Design review of the part built by this model. Coordinates are the model's own, in mm. Coordinates: 2 decimals unless noted, no trailing zeros. Write each loop counter-clockwise with the first axis right and the second up, starting at its lowest first coordinate (ties: lowest second). Pieces come first, ordered by that corner, then holes.
Q1. Take a section at B-B (y = -13.75). Give the boundary of the cut face in (x, z) (3 decimals), and give its area (3 significant figures).
Q2. Insertion check: pin 1 (10 mm diameter, centred on x = -0.5, y = -9.5, fed in from +Z). The pin has a flat end and moves straight along its axis. Give the tip position at first contact, or say it passes through.
Q3. Take a section at A-A (z = -18). Give the boundary of the cut face in (x, y) (3 decimals), and give its area (3 significant figures).
Q4. For probe 1 along X at (y, z) = (-3.5, 18) (3 decimals); probe 2 along Z at (x, y) = (0, -4); probe 3 along X at (y, z) = (-9.5, 34) (3 decimals), list the stretches that pass through material, from the lowest coordinate up.
Q5. Take a section at C-C (x = 0). Give the boundary of the cut face in (y, z).
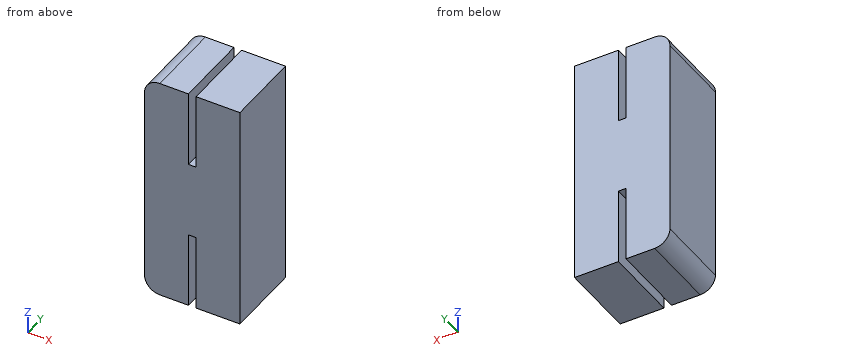
```python
from build123d import *

# Parameters (mm, degrees)
F0_W     = 31.75
F0_H     = 76.2
F1_DEPTH = 25.4
F2_W     = 2.54
F2_H     = 25.4
F3_DEPTH = 25.4
F4_R     = 5.08


with BuildPart() as f1:
    # F0 (on Front) → F1 (new body)
    with BuildSketch(Plane.XZ):
        Rectangle(F0_W, F0_H)
    extrude(amount=F1_DEPTH)

    # F2 (on face) → F3 (cut)
    with BuildSketch(Plane.XZ.offset(25.4)):
        with Locations((0, 25.4)):
            Rectangle(F2_W, F2_H)
        with Locations((0, -25.4)):
            Rectangle(F2_W, F2_H)
    extrude(amount=-F3_DEPTH, mode=Mode.SUBTRACT)

    # F4
    f4_edges = [f1.edges().sort_by_distance(p)[0] for p in [
        (-15.875, -12.7, 38.1),
        (-15.875, -12.7, -38.1),
    ]]
    fillet(f4_edges, radius=F4_R)


solid = f1.part
```
Response:
1. outline: (-15.875, -33.02) arc R5.08 ccw to (-10.795, -38.1) - (-1.27, -38.1) - (-1.27, -12.7) - (1.27, -12.7) - (1.27, -38.1) - (15.875, -38.1) - (15.875, 38.1) - (1.27, 38.1) - (1.27, 12.7) - (-1.27, 12.7) - (-1.27, 38.1) - (-10.795, 38.1) arc R5.08 ccw to (-15.875, 33.02) - close
1. area: 2,280 mm2
2. pin 1: stops at z = 38.1
3. outline: (-15.875, -25.4) - (-1.27, -25.4) - (-1.27, 0) - (-15.875, 0) - close; (1.27, -25.4) - (15.875, -25.4) - (15.875, 0) - (1.27, 0) - close
3. area: 742 mm2
4. probe 1: x = -15.875 to -1.27, 1.27 to 15.875
4. probe 2: z = -12.7 to 12.7
4. probe 3: x = -15.78 to -1.27, 1.27 to 15.875
5. outline: (-25.4, -12.7) - (0, -12.7) - (0, 12.7) - (-25.4, 12.7) - close
